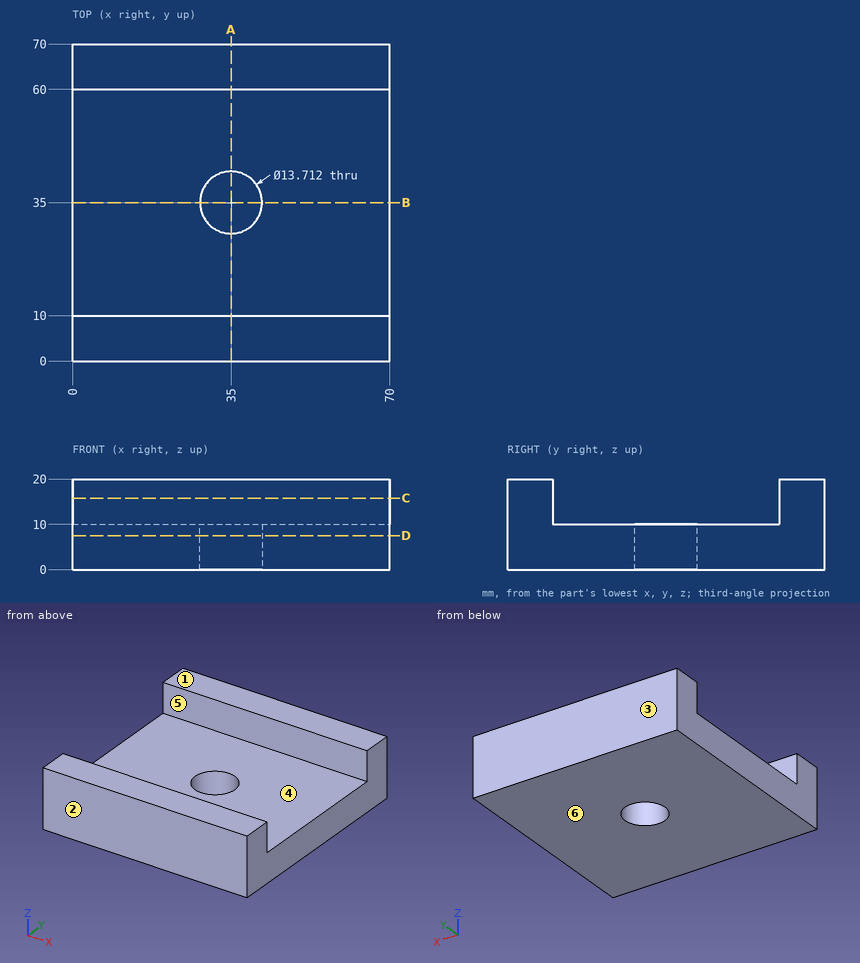
Geometry: see drawing. Coordinates: mm, zero at the bounding-box minimum. A direction names the side the tool comes from. Give positions to 0.01 mm unless a question says otherwise; leave off trailing zeros. Order: outer loops, then holes, each group sorted by start corner. A loop starts at its lowest first (then second) coordinate and runs counter-clockwise, first axis right, second up. Notation, with made-up numbers: (-27.75, -22) - (1.25, -22) arc R23 cw to (1.25, -11) - close; hole circle Ø1 at (80, 60.5). An arc over 180 degrees is marked (long way). Use CSV: the item, a comma, the result in double quotes.
1. Section query B-B (y = 35). Output: boundary loops of the cut face in (x, z), plus the area to 3 significant figures.
Answers below:
outline,"(0, 0) - (28.14, 0) - (28.14, 10) - (0, 10) - close; (41.86, 0) - (70, 0) - (70, 10) - (41.86, 10) - close"
area,"563 mm2"
2. Section query D-D (z = 7.5). Output: boundary loops of the cut face in (x, y).
Answers below:
outline,"(0, 0) - (70, 0) - (70, 70) - (0, 70) - close; hole circle Ø13.71 at (35, 35)"
3. Access query for the marked faces 5 and 6. Directions: +Z, -Z, +X, -X, +Y, -Y. A direction counts if a zero-diameter tool reaches every point of the face in a straight line with its end or side. Return the directions, or none.
Answers below:
face 5,"+Z, +X, -X"
face 6,"-Z, +X, -X, +Y, -Y"
4. Material intervals for line 1 along Y through (x, z) = (29, 13.25); line 2 along Y through (x, z) = (35, 3.75); line 3 along Z through (x, y) = (50, 35), sorted ascending. Write a range as from..to.
Answers below:
line 1,"0..10, 60..70"
line 2,"0..28.14, 41.86..70"
line 3,"0..10"
5. Section query C-C (z = 15.75). Output: boundary loops of the cut face in (x, y).
Answers below:
outline,"(0, 0) - (70, 0) - (70, 10) - (0, 10) - close; (0, 60) - (70, 60) - (70, 70) - (0, 70) - close"
6. Contact query for flat-ended pins moving along their axis: pin 1 (5 mm diameter, centred on x = 37, z = 13, fed in from -Y); pin 2 (18 mm diameter, centred on x = 35, y = 35, fed in from +Z); pin 3 (1 mm diameter, centred on y = 41.5, z = 11.5, fed in from -X). Output: stop coordinate, or through.
Answers below:
pin 1,"y = 0"
pin 2,"z = 10"
pin 3,"through"
7. Mould query, pull axis Y, two halves, no side actions, for the marked faces 1, 2, 3 and 4. Classes: +Y half, -Y half, draft (parallel to the pull), parting line (faces both ways), or undercut.
Answers below:
face 1,"draft"
face 2,"-Y half"
face 3,"+Y half"
face 4,"undercut"
8. Section query A-A (x = 35). Output: boundary loops of the cut face in (y, z).
Answers below:
outline,"(0, 0) - (28.14, 0) - (28.14, 10) - (10, 10) - (10, 20) - (0, 20) - close; (41.86, 0) - (70, 0) - (70, 20) - (60, 20) - (60, 10) - (41.86, 10) - close"
